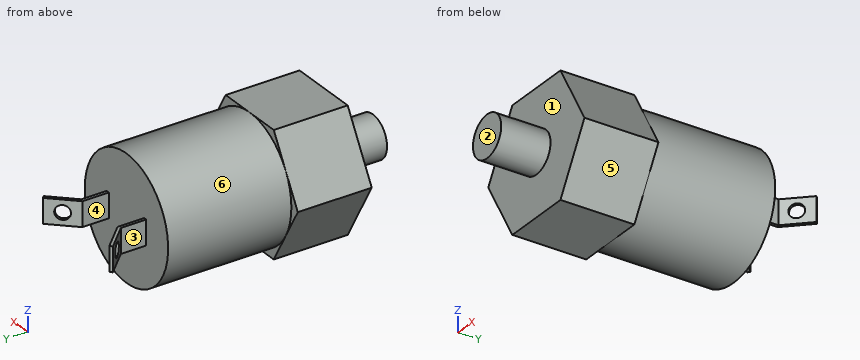
from build123d import *

# Parameters (mm, degrees)
BOSS_EXTRUDE1_DEPTH = 15.24
SKETCH3_R           = 12.7
BOSS_EXTRUDE2_DEPTH = 25.4
SKETCH4_R           = 4.3053
BOSS_EXTRUDE3_DEPTH = 10.16
EXTRUDE_THIN1_DEPTH = 2.54
SKETCH6_R           = 1.4605
CUT_EXTRUDE1_DEPTH  = 0.635


with BuildPart() as part:
    # Sketch2 → Boss-Extrude1 (new body)
    with BuildSketch(Plane(origin=(0, 0, 0), x_dir=(1, 0, 0), z_dir=(0, 1, 0))):
        Polygon((7.332348419, 12.7), (-7.332348419, 12.7), (-14.664696837, 0), (-7.332348419, -12.7), (7.332348419, -12.7), (14.664696837, 0), align=None)
    extrude(amount=BOSS_EXTRUDE1_DEPTH)

    # Sketch3 → Boss-Extrude2 (add)
    with BuildSketch(Plane(origin=(0, 15.24, 0), x_dir=(1, 0, 0), z_dir=(0, 1, 0))):
        Circle(SKETCH3_R)
    extrude(amount=BOSS_EXTRUDE2_DEPTH)

    # Sketch4 → Boss-Extrude3 (add)
    with BuildSketch(Plane.XZ):
        Circle(SKETCH4_R)
    extrude(amount=BOSS_EXTRUDE3_DEPTH)

    # Sketch5 → Extrude-Thin1 (add, symmetric)
    with BuildSketch(Plane.XY):
        Polygon((6.008182396, 40.64), (6.008182396, 45.866997676), (10.555270964, 50.579540341), (10.098307994, 51.020459659), (5.373182396, 46.123401761), (5.373182396, 40.64), align=None)
    extrude_thin1 = extrude(amount=EXTRUDE_THIN1_DEPTH, both=True)

    # Sketch6 → Cut-Extrude1 (cut)
    with BuildSketch(Plane(origin=(-20.264409117, 19.552939797, 0), x_dir=(0, 0, 1), z_dir=(-0.719626724, 0.69436113, 0))):
        with Locations((0, 40.325060137)):
            Circle(SKETCH6_R)
    cut_extrude1 = extrude(amount=-CUT_EXTRUDE1_DEPTH, mode=Mode.SUBTRACT)

    # Mirror1: Extrude-Thin1, Cut-Extrude1 across plane
    add(extrude_thin1.mirror(Plane(origin=(0, 0, 0), x_dir=(0, 0, 1), z_dir=(1, 0, 0))))
    add(cut_extrude1.mirror(Plane(origin=(0, 0, 0), x_dir=(0, 0, 1), z_dir=(1, 0, 0))), mode=Mode.SUBTRACT)


solid = part.part
The model under review builds one solid part; all positions refer to its coordinate system, in mm. Face numbers are marked on the shaded views. A direction names the side the tool comes from. Round coordinates to 2 decimals unless told otherwise and drop trailing zeros. Order: outer loops, then holes, each group sorted by start corner. A loop starts at its lowest first (then second) coordinate and runs counter-clockwise, first axis right, second up. Notation, with made-up numbers: (-32, -0.5) -> (21, -0.5) arc R15 ccw to (21, 26.5) -> close; hole circle Ø10 at (45.25, 50). An arc over 180 degrees is marked (long way). Return JSON: item names as keys, results as strings.
1. Insertion check: P1, Ø5.5, axis at y = 43.5, z = 0, coming from the +X side; P2, Ø4, axis at y = 42.5, z = -1, coming from the -X side; P3, Ø1.9, axis at x = -4.5, z = 8.5, coming from the +Y side. Each pin has a flat end and moves straight along its axis. Give the tip position at first contact, or say it passes through.
Answer block:
{"P1": "stops at x = 6.38", "P2": "stops at x = -12.7", "P3": "stops at y = 40.64"}
2. Take a section at D-D (y = 10). Write out the cut boundary in (x, z).
Answer block:
{"outline": "(-14.66, 0) -> (-7.33, -12.7) -> (7.33, -12.7) -> (14.66, 0) -> (7.33, 12.7) -> (-7.33, 12.7) -> close"}
3. The part is to be moulded in two halves that separate along X. For the marked faces 4, 5 and 6, say which applies: +X half, -X half, draft (parallel to the pull), parting line (faces both ways), or undercut.
Answer block:
{"face 4": "undercut", "face 5": "+X half", "face 6": "parting line"}
4. For L1, parallel to Z at x = 5.5, y = 43; L2, parallel to Y at x = -4.5, z = 7.5; L3, parallel to Y at x = -10.25, z = -1.75, list the stretches that pass through material, from the lowest coordinate up. Write a range as [from, to].
Answer block:
{"L1": "z = [-2.54, 2.54]", "L2": "y = [0, 40.64]", "L3": "y = [0, 40.64], [50.26, 50.87]"}
5. Take a section at A-A (y = 43). Write out the cut boundary in (x, z).
Answer block:
{"outline": "(-6.01, -2.54) -> (-5.37, -2.54) -> (-5.37, 2.54) -> (-6.01, 2.54) -> close; (5.37, -2.54) -> (6.01, -2.54) -> (6.01, 2.54) -> (5.37, 2.54) -> close"}
6. For the marked faces 1, 2 and 3, list the 3-axis set-ups (+Z, -Z, +X, -X, +Y, -Y) from which the entire face can be reached by the end or side of a thin tool; tool diameter is ignored.
Answer block:
{"face 1": "-Y", "face 2": "+Z, -Z, +X, -X, -Y", "face 3": "+Z, -Z, -X"}
7. Take a section at B-B (y = 28.5). Write out the cut boundary in (x, z).
Answer block:
{"outline": "circle Ø25.4 at (0, 0)"}
8. Take a section at C-C (z = -5.5). Write out the cut boundary in (x, y).
Answer block:
{"outline": "(-11.49, 0) -> (11.49, 0) -> (11.49, 15.24) -> (11.45, 15.24) -> (11.45, 40.64) -> (-11.45, 40.64) -> (-11.45, 15.24) -> (-11.49, 15.24) -> close"}
